Part model, mm, in its own coordinate system. A direction names the side the tool comes from. Round coordinates to 2 decimals unless told otherwise and drop trailing zeros. Loops run counter-clockwise (first coordinate to the right, second up) from the corner with the lowest first, then second, coordinate; pieces in that order, holes last.
(1) Probe probe 1 along X at (y, z) = (16.5, 7.5); probe 2 along Z at (x, y) = (78.5, 6.5); probe 3 along Z at (x, y) = (43, 4.5). List the from-to ranges inside material, lowest first.
(2) Cut at D-D on y = 13.25. List the corners of the cut face in (x, z) (3 decimals), then the cut area to 4 significant figures.
(3) Flat gauge pins, fed straight in: pin 1 (5 mm diameter, centred on x = 17, z = -47, fed in from -Y); pin 2 (4 mm diameter, centred on x = 40, y = 4.5, fed in from -Z); pin 3 (14 mm diameter, centred on y = 14.5, z = -22, fed in from +X); pin 4 (5 mm diameter, centred on x = 78, y = 10, fed in from -Z). Where does each tip first touch, or does it go through?
(4) Cut at B-B on z = -81. List the corners of the cut face in (x, y), then the cut area to 3 significant figures.
(5) Tool access for faces 5 (the face through (100, 14, -64)), 6 (the face through (53.244, 19.621, 27.414)): list every direction of +Z, -Z, +X, -X, +Y, -Y with a clear straight run to the whole face (end or side of a thin tool).
(6) Mould opens along Z. For faces 1 (the face through (53, 25, -160)), 2 (the face through (108, 28.2, -65.8)), 3 (the face through (104, 22, -158)), 4 (the face through (49.3, 8.715, 13.073)) say: +Z half, -Z half, draft (parallel to the pull), parting line (faces both ways), or undercut.
(7) Cut at A-A on x = 51. List the corners of the cut face in (y, z).
(8) Cut at C-C on y = 25. List the corners of the cut face in (x, z), then the cut area to 3 significant figures.
Autodesk Inventor part; units mm, degrees
ref_plane "YZ Plane" through (0, 0, 0) normal (1, 0, 0) x (0, 1, 0)
ref_plane "XZ Plane" through (0, 0, 0) normal (0, 1, 0) x (-1, 0, 0)
ref_plane "XY Plane" through (0, 0, 0) normal (0, 0, 1) x (1, 0, 0)
sketch "Sketch1" plane through (0, 0, 0) normal (1, 0, 0) x (0, 1, 0)
  line L0 (0, 0) -> (0, -150)
  line L1 (20, -160) -> (0, -150)
  line L2 (30, 0) -> (21.3239, 26.0284)
  arc A0 (21.3239, 26.0284) -> (17.6778, 26.5166) centre (19.3814, 25.3809) ccw
  line L3 (0, 0) -> (17.6778, 26.5166)
  line L4 (20, -160) -> (30, -160)
  line L5 (30, -160) -> (30, 0)
  dimension "d0" = 150
  dimension "d4" = 30
extrude "Extrusion1" add sketch "Sketch1" along normal blind 100
sketch "Sketch2" plane through (100, 0, 0) normal (1, 0, 0) x (0, 0, -1)
  line L0 (0, 30) -> (160, 30)
  line L1 (160, 30) -> (160, 20)
  line L2 (0, 30) -> (-26.0284, 21.3239)
  line L3 (0, 30) -> (-26.0284, 21.3239)
  arc A0 (-26.0284, 21.3239) -> (-26.5166, 17.6778) centre (-25.3809, 19.3814) ccw
  arc A1 (-26.0284, 21.3239) -> (-27.3197, 18.7231) centre (-25.3809, 19.3814) ccw
  line L4 (160, 20) -> (160, 30)
  line L5 (158, 28) -> (0, 28)
  line L6 (0, 28) -> (-25.3809, 19.3814)
  line L7 (-25.3809, 19.3814) -> (-27.4284, 18.6861)
  line L8 (158, 28) -> (158, 16)
  line L9 (150, 0) -> (160, 20)
  line L10 (160, 20) -> (158, 16)
  point P0 (0, 0)
  dimension "d7" = 2
extrude "Extrusion2" add sketch "Sketch2" along normal blind 8
sketch "Sketch3" plane through (0, 30, 0) normal (0, 1, 0) x (1, 0, 0)
  point P0 (0, 0)
properties part number "Tank body"
Final values:
1. probe 1: x = 0 to 100
1. probe 2: z = -153.25 to 9.75
1. probe 3: z = -152.25 to 6.75
2. outline: (0, -156.625) - (100, -156.625) - (100, 19.875) - (0, 19.875) - close
2. area: 17,650 mm2
3. pin 1: stops at y = 0
3. pin 2: stops at z = -153.25
3. pin 3: stops at x = 100
3. pin 4: stops at z = -156.25
4. outline: (0, 0) - (100, 0) - (100, 28) - (108, 28) - (108, 30) - (0, 30) - close
4. area: 3,020 mm2
5. face 5: +X, -Y
5. face 6: +Z, +X, -X
6. face 1: -Z half
6. face 2: draft
6. face 3: undercut
6. face 4: +Z half
7. outline: (0, -150) - (20, -160) - (30, -160) - (30, 0) - (21.32, 26.03) arc R2.05 ccw to (17.68, 26.52) - (0, 0) - close
8. outline: (0, -160) - (108, -160) - (108, -158) - (100, -158) - (100, 8.83) - (108, 8.83) - (108, 15) - (0, 15) - close
8. area: 17,600 mm2
